Build history of the part. All positions in model axes, mm. A direction names the side the tool comes from. Round coordinates to 2 decimals unless told otherwise and drop trailing zeros. Write each loop counter-clockwise with the first axis right and the second up, starting at its lowest first coordinate (ties: lowest second). Pieces come first, ordered by that corner, then holes.
Autodesk Inventor part; units mm, degrees
ref_plane "YZ Plane" through (0, 0, 0) normal (1, 0, 0) x (0, 1, 0)
ref_plane "XZ Plane" through (0, 0, 0) normal (0, 1, 0) x (-1, 0, 0)
ref_plane "XY Plane" through (0, 0, 0) normal (0, 0, 1) x (1, 0, 0)
sketch "Sketch1" plane through (0, 0, 0) normal (0, 0, 1) x (1, 0, 0)
  line L0 (-16.3, 0) -> (97.8, 0) construction
  line L1 (0, 210) -> (0, -210) construction
  line L2 (65.5, -150) -> (65.5, 150)
  line L3 (65.5, 150) -> (67.5, 150)
  line L4 (81.5, -147) -> (81.5, -150)
  line L5 (81.5, -150) -> (65.5, -150)
  line L6 (67.5, -142) -> (67.5, 142)
  line L7 (81.5, -147) -> (72.5, -147)
  line L8 (72.5, -147) -> (67.5, -142)
  line L9 (81.5, 150) -> (65.5, 150)
  line L10 (81.5, 150) -> (81.5, 147)
  line L11 (81.5, 147) -> (72.5, 147)
  line L12 (72.5, 147) -> (67.5, 142)
  point P0 (0, 0)
  dimension "d0" = 300
  dimension "d5" = 81.5
  dimension "d6" = 2
  dimension "d7" = 9
  dimension "d8" = 5
  dimension "d9" = 45
  dimension "d10" = 16
  dimension "d11" = 3
  dimension "d12" = 3
  dimension "d13" = 9
  dimension "d14" = 45
  dimension "d15" = 5
revolve "Revolution1" add sketch "Sketch1" angle 360 about axis through (0, 0, 0) along (0, -1, 0)
sketch "Sketch2" plane through (0, -150, 0) normal (0, -1, 0) x (1, 0, 0)
  line L0 (0, 114.1) -> (0, -114.1) construction
  line L1 (-114.1, 0) -> (114.1, 0) construction
  circle A0 centre (0, 0) radius 81.5 construction
  circle A1 centre (0, 0) radius 65.5 construction
  circle A2 centre (0, 0) radius 77 construction
  circle A3 centre (0, 0) radius 72.5 construction
  point P0 (0, 77)
  point P1 (-66.684, 38.5)
  point P2 (-66.684, -38.5)
  point P3 (0, -77)
  point P4 (66.684, -38.5)
  point P5 (66.684, 38.5)
  dimension "d16" = 4.5
  dimension "d20" = 360
  dimension "d29" = 4.5
hole "Hole1" at (0, -150, 77) at (-66.684, -150, 38.5) at (-66.684, -150, -38.5) at (0, -150, -77) at (66.684, -150, -38.5) at (66.684, -150, 38.5) direction (0, 1, 0) diameter 4.5 depth 13 tip angle 118
mirror "Mirror1" about plane through (0, 0, 0) normal (0, 1, 0) of "Hole1"
equation "\"d16\" = d29"
equation "\"d12\" = d11"
equation "\"d13\" = d7"
equation "\"d14\" = d9"
equation "\"d15\" = d8"
properties part number "Link_2" material "Aluminum 6061"
1) Slice it at A-A (z = 0). Write the cut outline in (x, y).
Results:
outline: (-81.5, -150) - (-65.5, -150) - (-65.5, 150) - (-81.5, 150) - (-81.5, 147) - (-72.5, 147) - (-67.5, 142) - (-67.5, -142) - (-72.5, -147) - (-81.5, -147) - close; (65.5, -150) - (81.5, -150) - (81.5, -147) - (72.5, -147) - (67.5, -142) - (67.5, 142) - (72.5, 147) - (81.5, 147) - (81.5, 150) - (65.5, 150) - close
2) Mould opens along Y. For faces 1 (the cylindrical face through (62.475, 2.1, -19.674)), 2 (the conical face through (-14.7, -142.31, -66.2)), 3 (the flat face through (-61, 150, 25)) say: released by +Y, released by -Y, zero draft, split by the parting line, or undercut.
Results:
face 1: zero draft
face 2: undercut
face 3: released by +Y
3) Pin check, flat tips, straight feed: pin 1 Ø1 at (y, z) = (-60.5, -10) entering from -X; pin 2 Ø1 at (y, z) = (81, -1.5) entering from +X; pin 3 Ø6 at (x, z) = (0, -77) entering from -Y; pin 4 Ø5 at (x, y) = (31.5, -83) entering from +Z. Stop position of each tip, or through.
Results:
pin 1: stops at x = -66.83
pin 2: stops at x = 67.49
pin 3: stops at y = -150
pin 4: stops at z = 60.95
4) Slice it at B-B (y = -4). Write the cut outline in (x, z), plus the area to 3 significant figures.
Results:
outline: circle Ø135 at (0, 0); hole circle Ø131 at (0, 0)
area: 836 mm2
5) Which spindle directions (+Z, -Z, +X, -X, +Y, -Y) get a long thin tool onto all of the face, cutting with end or side? Do faces 4 (the flat face through (-61, -150, 25)), 5 (the conical face through (-14.7, 142.31, 66.2)). Say none if no direction does.
Results:
face 4: +Z, -Z, +X, -X, -Y
face 5: none
6) Wall check: L1, parallel to Y at x = -69, z = -34.5; L2, parallel to Z at x = 0, y = 24; L3, parallel to X at y = 102, z = 6. Give the ranges that are in metal, low to high.
Results:
L1: y = -150 to -147, 147 to 150
L2: z = -67.5 to -65.5, 65.5 to 67.5
L3: x = -67.23 to -65.22, 65.22 to 67.23
